```python
from build123d import *

# Parameters (mm, degrees)
PATTERN_CIRCULAR_2_COUNT = 6
SKETCH_8_R               = 2
CUT_EXTRUDE_1_DEPTH      = 3.7
PATTERN_CIRCULAR_3_COUNT = 3
CHAMFER_1_SIZE           = 0.3
CHAMFER_3_SIZE           = 0.3
EXTRUDE_START            = 0.3
SKETCH_12_R              = 3
SKETCH_12_R_2            = 2
EXTRUDE_1_DEPTH          = 0.3
CHAMFER_4_SIZE           = 0.3
EXTRUDE_START_2          = 3
SKETCH_13_R              = 0.785
EXTRUDE_2_DEPTH          = 3
CHAMFER_5_SIZE           = 0.3
SKETCH_14_R              = 0.75
CUT_EXTRUDE_2_DEPTH      = 24.775828061


with BuildPart() as part:
    # 草图1 → 旋转1 (revolve)
    with BuildSketch(Plane.XY, mode=Mode.PRIVATE) as revolve_1_sk:
        Polygon((16, 3), (15, 3), (15, 8), (6.5, 8), (6.5, 4), (5.5, 4), (5.5, 3), (0.785, 3), (0.785, 0), (15, 0), (15, 2), (16, 2), align=None)
    revolve(revolve_1_sk.sketch.rotate(Axis((0, 0, 0), (0, -1, 0)), 90), axis=Axis((0, 0, 0), (0, -1, 0)))

    # 草图7 → M3 螺纹孔2 (revolve, cut)
    with BuildSketch(Plane(origin=(-12, 0, 0), x_dir=(0, 0, -1), z_dir=(1, 0, 0))):
        Polygon((0, 0), (0, 7.5), (1.25, 6.748924226), (1.25, 0), align=None)
    hole_wizard_m3_2 = revolve(axis=Axis((-12, -6.35, 0), (0, 1, 0)), mode=Mode.SUBTRACT)

    # 阵列(圆周)2: M3 螺纹孔2 ×6 about axis
    pattern_circular_2_axis = Axis((0, 0, 0), (0, 1, 0))
    for i in range(1, PATTERN_CIRCULAR_2_COUNT):
        add(hole_wizard_m3_2.rotate(pattern_circular_2_axis, i * 360 / PATTERN_CIRCULAR_2_COUNT), mode=Mode.SUBTRACT)

    # 草图8 → 切除-拉伸1 (cut)
    with BuildSketch(Plane(origin=(0, 8, 0), x_dir=(1, 0, 0), z_dir=(0, 1, 0))):
        with Locations(Location((0, 10.59, 0), (0, 0, 270))):
            Circle(SKETCH_8_R)
    cut_extrude_1 = extrude(amount=-CUT_EXTRUDE_1_DEPTH, mode=Mode.SUBTRACT)

    # 阵列(圆周)3: 切除-拉伸1 ×3 about axis
    pattern_circular_3_axis = Axis((0, 0, 0), (0, 1, 0))
    for i in range(1, PATTERN_CIRCULAR_3_COUNT):
        add(cut_extrude_1.rotate(pattern_circular_3_axis, i * 360 / PATTERN_CIRCULAR_3_COUNT), mode=Mode.SUBTRACT)

    # 倒角1
    chamfer_1_edges = [part.edges().sort_by_distance(p)[0] for p in [
        (0, 0, -15),
        (0, 8, -15),
        (0, 8, -6.5),
    ]]
    chamfer(chamfer_1_edges, length=CHAMFER_1_SIZE)

    # 倒角3
    chamfer_3_edges = [part.edges().sort_by_distance(p)[0] for p in [
        (0, 3, -0.785),
    ]]
    chamfer(chamfer_3_edges, length=CHAMFER_3_SIZE)

    # 草图12 → 凸台-拉伸1 (add)
    # profile 1 of 3: a face of its own
    with BuildSketch(Plane(origin=(0, 8, 0), x_dir=(1, 0, 0), z_dir=(0, 1, 0)).offset(EXTRUDE_START)):
        with Locations(Location((0, 10.59, 0), (0, 0, 90))):
            Circle(SKETCH_12_R)
        with Locations(Location((0, 10.59, 0), (0, 0, 270))):
            Circle(SKETCH_12_R_2, mode=Mode.SUBTRACT)
    # profile 2 of 3: a face of its own
    with BuildSketch(Plane(origin=(0, 8, 0), x_dir=(1, 0, 0), z_dir=(0, 1, 0)).offset(EXTRUDE_START)):
        with Locations(Location((-9.171209026, -5.295, 0), (0, 0, 90))):
            Circle(SKETCH_12_R)
        with Locations(Location((-9.171209026, -5.295, 0), (0, 0, 270))):
            Circle(SKETCH_12_R_2, mode=Mode.SUBTRACT)
    # profile 3 of 3: a face of its own
    with BuildSketch(Plane(origin=(0, 8, 0), x_dir=(1, 0, 0), z_dir=(0, 1, 0)).offset(EXTRUDE_START)):
        with Locations(Location((9.171209026, -5.295, 0), (0, 0, 90))):
            Circle(SKETCH_12_R)
        with Locations(Location((9.171209026, -5.295, 0), (0, 0, 270))):
            Circle(SKETCH_12_R_2, mode=Mode.SUBTRACT)
    extrude(amount=-EXTRUDE_1_DEPTH)

    # 倒角4
    # the kernel refuses this chamfer: 0.3 mm, written as the material it takes off along each edge
    with BuildSketch(Plane(origin=(9.171209026, 8.3, 5.295), x_dir=(0, 0, 1), z_dir=(-1, 0, 0))) as chamfer_4_piece_1:
        Polygon((2 + CHAMFER_4_SIZE, 0), (2, -CHAMFER_4_SIZE), (2, 0), align=None)
    revolve(axis=Axis((9.171209026, 8.3, 5.295), (0, 1, 0)), mode=Mode.SUBTRACT)
    with BuildSketch(Plane(origin=(0, 8.3, -10.59), x_dir=(0, 0, 1), z_dir=(-1, 0, 0))) as chamfer_4_piece_2:
        Polygon((2 + CHAMFER_4_SIZE, 0), (2, -CHAMFER_4_SIZE), (2, 0), align=None)
    revolve(axis=Axis((0, 8.3, -10.59), (0, 1, 0)), mode=Mode.SUBTRACT)
    with BuildSketch(Plane(origin=(-9.171209026, 8.3, 5.295), x_dir=(0, 0, 1), z_dir=(-1, 0, 0))) as chamfer_4_piece_3:
        Polygon((2 + CHAMFER_4_SIZE, 0), (2, -CHAMFER_4_SIZE), (2, 0), align=None)
    revolve(axis=Axis((-9.171209026, 8.3, 5.295), (0, 1, 0)), mode=Mode.SUBTRACT)

    # 草图13 → 凸台-拉伸2 (add)
    with BuildSketch(Plane.XZ.offset(EXTRUDE_START_2)):
        with BuildLine():
            Line((-3, 6.92820323), (-3, -6.92820323))
            ThreePointArc((-3, -6.92820323), (-2.511857892, -8.237510572), (-1.285714286, -8.907689867))
            ThreePointArc((-1.285714286, -8.907689867), (0, -9), (1.285714286, -8.907689867))
            ThreePointArc((1.285714286, -8.907689867), (2.511857892, -8.237510572), (3, -6.92820323))
            Line((3, -6.92820323), (3, 6.92820323))
            ThreePointArc((3, 6.92820323), (2.511857892, 8.237510572), (1.285714286, 8.907689867))
            ThreePointArc((1.285714286, 8.907689867), (0, 9), (-1.285714286, 8.907689867))
            ThreePointArc((-1.285714286, 8.907689867), (-2.511857892, 8.237510572), (-3, 6.92820323))
        make_face()
        with Locations(Location((0, 0, 0), (0, 0, 270))):
            Circle(SKETCH_13_R, mode=Mode.SUBTRACT)
    extrude(amount=-EXTRUDE_2_DEPTH)

    # 倒角5
    chamfer_5_edges = [part.edges().sort_by_distance(p)[0] for p in [
        (-2.511857892, -3, -8.237510572),
        (0, -3, -9),
        (2.511857892, -3, -8.237510572),
        (3, -3, 0),
        (2.511857892, -3, 8.237510572),
        (0, -3, 9),
        (-2.511857892, -3, 8.237510572),
        (-3, -3, 0),
    ]]
    chamfer(chamfer_5_edges, length=CHAMFER_5_SIZE)

    # 草图14 → 切除-拉伸2 (cut, through all)
    with BuildSketch(Plane(origin=(0, 4.3, 0), x_dir=(1, 0, 0), z_dir=(0, 1, 0))):
        with Locations(Location((9.171209026, -5.295, 0), (0, 0, 270))):
            Circle(SKETCH_14_R)
        with Locations(Location((0, 10.59, 0), (0, 0, 270))):
            Circle(SKETCH_14_R)
        with Locations(Location((-9.171209026, -5.295, 0), (0, 0, 270))):
            Circle(SKETCH_14_R)
    extrude(amount=-CUT_EXTRUDE_2_DEPTH, mode=Mode.SUBTRACT)


solid = part.part
```
Geometry: final body of the model. Coordinates: model frame, mm. A direction names the side the tool comes from. Coordinates: 2 decimals unless noted, no trailing zeros. Order: outer loops, then holes, each group sorted by start corner. A loop starts at its lowest first (then second) coordinate and runs counter-clockwise, first axis right, second up. Notation, with made-up numbers: M 80,16 L 135,16 A12 cw 135,26 Z; hole C 81,10.5 d8. An arc over 180 degrees is marked long. Answer in a Markdown table with one row per item. Add a question column.
Q1. Section query A-A on y = -1. Return the cut outline in (x, z) (3 decimals).
Q2. Mould query, pull axis Z, two halves, no side actions, for faces 1 (the cylindrical face through (0, -1, -9)), 2 (the flat face through (-3.5, 0, 0.2)), 3 (the conical face through (5.82, 7.37, -10.51)), 4 (the flat face through (-8, 4.3, 5)). Classes: released by +Z, released by -Z, zero draft, split by the parting line, or undercut.
Q3. Reachability of faces 5 (the cylindrical face through (6.479, 3.327, -11.547)), 6 (the cylindrical face through (-2.5, -1.37, 8.25)), 7 (the cylindrical face through (-7.82, 6.18, 3.82)) from +Z, -Z, +X, -X, +Y, -Y: full face, straight path, thin tool, end or side. Return the list, or none.
Q4. Section query B-B on y = 5. Count the separate pieces of the cut face and the enclosed holes in it, and give its area (3 significant figures).
Q5. Line query: L1, parallel to X at y = -1.8, z = 0 (3 decimals); L2, parallel to Z at x = -5.5, y = 0.75; L3, parallel to X at y = 1.3, z = -10.59. Output: solid intervals per line, ascending.
Q6. Contact query for flat-ended pins moving along their axis: P1, Ø10, axis at x = 12, z = 10, coming from the -Y side; P2, Ø1.4, axis at y = -1.5, z = 1, coming from the +X side; P3, Ø2, axis at x = 6.5, y = 4.5, coming from the -Z side; P4, Ø1, axis at x = -8, y = -1.5, coming from the +Z side. Output: stop coordinate, or through.
Completed:
| question | item | result |
|---|---|---|
| 1 | outline | M -3,-6.928 A2 ccw -1.286,-8.908 A9 ccw 1.286,-8.908 A2 ccw 3,-6.928 L 3,6.928 A2 ccw 1.286,8.908 A9 ccw -1.286,8.908 A2 ccw -3,6.928 Z; hole C 0,0 d1.57 |
| 2 | face 1 | released by -Z |
| 2 | face 2 | zero draft |
| 2 | face 3 | undercut |
| 2 | face 4 | undercut |
| 3 | face 5 | -Y |
| 3 | face 6 | +Z, -X, -Y |
| 3 | face 7 | +Y |
| 4 | separate pieces | 1 |
| 4 | enclosed holes | 10 |
| 4 | area | 507 mm2 |
| 5 | L1 | x = -3 to -0.785, 0.785 to 3 |
| 5 | L2 | z = -13.96 to -11.54, -9.25 to 9.25, 11.54 to 13.96 |
| 5 | L3 | x = -10.62 to -7.23, -4.77 to -0.75, 0.75 to 4.77, 7.23 to 10.62 |
| 6 | P1 | stops at y = 0 |
| 6 | P2 | stops at x = 3 |
| 6 | P3 | stops at z = -13.96 |
| 6 | P4 | passes through |
